```python
from build123d import *

# Parameters (mm, degrees)
BOSS_EXTRUDE1_DEPTH = 12


with BuildPart() as part:
    # Sketch1 → Boss-Extrude1 (new body)
    with BuildSketch(Plane.XY):
        with BuildLine():
            Line((562.664353911, 109.833333333), (553.064353911, 109.833333333))
            ThreePointArc((553.064353911, 109.833333333), (548.967297637, 111.530389608), (550.664353911, 107.433333333))
            Line((550.664353911, 107.433333333), (550.664353911, 76.233333333))
            ThreePointArc((550.664353911, 76.233333333), (548.967297637, 72.136277058), (553.064353911, 73.833333333))
            Line((553.064353911, 73.833333333), (562.664353911, 73.833333333))
            Line((562.664353911, 73.833333333), (562.664353911, 37.833333333))
            Line((562.664353911, 37.833333333), (553.064353911, 37.833333333))
            ThreePointArc((553.064353911, 37.833333333), (548.967297637, 39.530389608), (550.664353911, 35.433333333))
            Line((550.664353911, 35.433333333), (550.664353911, 4.233333333))
            ThreePointArc((550.664353911, 4.233333333), (548.967297637, 0.136277058), (553.064353911, 1.833333333))
            Line((553.064353911, 1.833333333), (562.664353911, 1.833333333))
            Line((562.664353911, 1.833333333), (562.664353911, -34.166666667))
            Line((562.664353911, -34.166666667), (553.064353911, -34.166666667))
            ThreePointArc((553.064353911, -34.166666667), (548.967297637, -32.469610392), (550.664353911, -36.566666667))
            Line((550.664353911, -36.566666667), (550.664353911, -67.766666667))
            ThreePointArc((550.664353911, -67.766666667), (548.967297637, -71.863722942), (553.064353911, -70.166666667))
            Line((553.064353911, -70.166666667), (562.664353911, -70.166666667))
            Line((562.664353911, -70.166666667), (562.664353911, -106.166666667))
            Line((562.664353911, -106.166666667), (553.064353911, -106.166666667))
            ThreePointArc((553.064353911, -106.166666667), (548.967297637, -104.469610392), (550.664353911, -108.566666667))
            Line((550.664353911, -108.566666667), (550.664353911, -139.766666667))
            ThreePointArc((550.664353911, -139.766666667), (548.967297637, -143.863722942), (553.064353911, -142.166666667))
            Line((553.064353911, -142.166666667), (562.664353911, -142.166666667))
            Line((562.664353911, -142.166666667), (562.664353911, -178.166666667))
            Line((562.664353911, -178.166666667), (553.064353911, -178.166666667))
            ThreePointArc((553.064353911, -178.166666667), (548.967297637, -176.469610392), (550.664353911, -180.566666667))
            Line((550.664353911, -180.566666667), (550.664353911, -211.766666667))
            ThreePointArc((550.664353911, -211.766666667), (548.967297637, -215.863722942), (553.064353911, -214.166666667))
            Line((553.064353911, -214.166666667), (562.664353911, -214.166666667))
            Line((562.664353911, -214.166666667), (562.664353911, -250.166666667))
            Line((562.664353911, -250.166666667), (-562.335646089, -250.166666667))
            Line((-562.335646089, -250.166666667), (-562.335646089, -214.166666667))
            Line((-562.335646089, -214.166666667), (-552.735646089, -214.166666667))
            ThreePointArc((-552.735646089, -214.166666667), (-548.638589814, -215.863722942), (-550.335646089, -211.766666667))
            Line((-550.335646089, -211.766666667), (-550.335646089, -180.566666667))
            ThreePointArc((-550.335646089, -180.566666667), (-548.638589814, -176.469610392), (-552.735646089, -178.166666667))
            Line((-552.735646089, -178.166666667), (-562.335646089, -178.166666667))
            Line((-562.335646089, -178.166666667), (-562.335646089, -142.166666667))
            Line((-562.335646089, -142.166666667), (-552.735646089, -142.166666667))
            ThreePointArc((-552.735646089, -142.166666667), (-548.638589814, -143.863722942), (-550.335646089, -139.766666667))
            Line((-550.335646089, -139.766666667), (-550.335646089, -108.566666667))
            ThreePointArc((-550.335646089, -108.566666667), (-548.638589814, -104.469610392), (-552.735646089, -106.166666667))
            Line((-552.735646089, -106.166666667), (-562.335646089, -106.166666667))
            Line((-562.335646089, -106.166666667), (-562.335646089, -70.166666667))
            Line((-562.335646089, -70.166666667), (-552.735646089, -70.166666667))
            ThreePointArc((-552.735646089, -70.166666667), (-548.638589814, -71.863722942), (-550.335646089, -67.766666667))
            Line((-550.335646089, -67.766666667), (-550.335646089, -36.566666667))
            ThreePointArc((-550.335646089, -36.566666667), (-548.638589814, -32.469610392), (-552.735646089, -34.166666667))
            Line((-552.735646089, -34.166666667), (-562.335646089, -34.166666667))
            Line((-562.335646089, -34.166666667), (-562.335646089, 1.833333333))
            Line((-562.335646089, 1.833333333), (-552.735646089, 1.833333333))
            ThreePointArc((-552.735646089, 1.833333333), (-548.638589814, 0.136277058), (-550.335646089, 4.233333333))
            Line((-550.335646089, 4.233333333), (-550.335646089, 35.433333333))
            ThreePointArc((-550.335646089, 35.433333333), (-548.638589814, 39.530389608), (-552.735646089, 37.833333333))
            Line((-552.735646089, 37.833333333), (-562.335646089, 37.833333333))
            Line((-562.335646089, 37.833333333), (-562.335646089, 73.833333333))
            Line((-562.335646089, 73.833333333), (-552.735646089, 73.833333333))
            ThreePointArc((-552.735646089, 73.833333333), (-548.638589814, 72.136277058), (-550.335646089, 76.233333333))
            Line((-550.335646089, 76.233333333), (-550.335646089, 107.433333333))
            ThreePointArc((-550.335646089, 107.433333333), (-548.638589814, 111.530389608), (-552.735646089, 109.833333333))
            Line((-552.735646089, 109.833333333), (-562.335646089, 109.833333333))
            Line((-562.335646089, 109.833333333), (-562.335646089, 145.833333333))
            Line((-562.335646089, 145.833333333), (562.664353911, 145.833333333))
            Line((562.664353911, 145.833333333), (562.664353911, 109.833333333))
        make_face()
    extrude(amount=BOSS_EXTRUDE1_DEPTH)


solid = part.part
```
Input: part model. Units: mm. Frame: model coordinates. Give positions to 0.01 mm unless a question says otherwise; leave off trailing zeros. Order: outer loops, then holes, each group sorted by start corner. A loop starts at its lowest first (then second) coordinate and runs counter-clockwise, first axis right, second up. Notation, with made-up numbers: M 67,-7.75 L 121,-7.75 A9 cw 121,-0.75 Z; hole C 88,17.5 d11. An arc over 180 degrees is marked long. Return JSON: item names as keys, results as strings.
Item 1: Ray query, probe 1 along X at (y, z) = (24.5, 11). Return the intervals inside material, ascending.
Solutions:
{"probe 1": "-550.34 to 550.66"}
Item 2: First-contact query: P1, Ø6, axis at y = 32.5, z = 7.5, coming from the -X side; P2, Ø4, axis at x = -550.34, y = -106.17, coming from the -Z side. Flat tips, straight axial feed; report the tip coordinate or a pass-through.
Solutions:
{"P1": "x = -550.34", "P2": "through"}
Item 3: Cut plane A-A (y = -53). Return loops of the section in (x, z), then the cut area to 3 significant figures.
Solutions:
{"outline": "M -550.34,0 L 550.66,0 L 550.66,12 L -550.34,12 Z", "area": "13,200 mm^2"}
